from build123d import *

# Parameters (mm, degrees)
F0_R          = 7
F1_DEPTH      = 45
F4_DEPTH      = 10.5
F4_DEPTH_BACK = 13.5


with BuildPart() as f1:
    # F0 (on Front) → F1 (new body)
    with BuildSketch(Plane.XZ):
        with BuildLine():
            Line((-33.5, 28.5), (-40.5, 21.5))
            Line((-40.5, 21.5), (-40.5, -6.2290436868))
            Line((-40.5, -6.2290436868), (-32.4062898078, -13.2290436868))
            Line((-32.4062898078, -13.2290436868), (-4.3396635525, -13.2290436868))
            ThreePointArc((-4.3396635525, -13.2290436868), (-1.1020136669, -14.4188437946), (0.5947737455, -17.4219943993))
            ThreePointArc((0.5947737455, -17.4219943993), (2.6248372639, -24.3164832501), (6.2880673968, -30.5))
            Line((6.2880673968, -30.5), (14.5, -30.5))
            Line((14.5, -30.5), (43.5, 4.5))
            Line((43.5, 4.5), (43.5, 23.5))
            Line((43.5, 23.5), (35.5, 28.5))
            Line((35.5, 28.5), (6.5, 28.5))
            ThreePointArc((6.5, 28.5), (-0.361821699, 25.4052447636), (-7.8869164215, 25.2180111709))
            Line((-7.8869164215, 25.2180111709), (-26.5, 28.5))
            Line((-26.5, 28.5), (-33.5, 28.5))
        make_face()
        with Locations((-26.5, 0.7709563132)):
            Circle(F0_R, mode=Mode.SUBTRACT)
    extrude(amount=F1_DEPTH)

    # F3 (on offset) → F4 (cut, two sides)
    with BuildSketch(Plane.XZ.offset(22.5)) as f4_sk:
        with BuildLine():
            Line((35.5, 28.5), (11.6408265143, 28.5))
            ThreePointArc((11.6408265143, 28.5), (17.6190851715, 7.4683040803), (33.5571428571, -7.5))
            Line((33.5571428571, -7.5), (43.5, 4.5))
            Line((43.5, 4.5), (43.5, 23.5))
            Line((43.5, 23.5), (35.5, 28.5))
        make_face()
    extrude(amount=-F4_DEPTH, mode=Mode.SUBTRACT)
    extrude(f4_sk.sketch, amount=F4_DEPTH_BACK, mode=Mode.SUBTRACT)


solid = f1.part
The model under review builds one solid part; all positions refer to its coordinate system, in mm. A direction names the side the tool comes from. Coordinates: 2 decimals unless noted, no trailing zeros. Loops run counter-clockwise (first coordinate to the right, second up) from the corner with the lowest first, then second, coordinate; pieces in that order, holes last.
(1) Consider section C-C, the plane z = 16. Give the boundary of the cut face in (x, y), plus the area to 3 significant figures.
Determined:
outline: (-40.5, -45) - (43.5, -45) - (43.5, -36) - (13.69, -36) - (13.69, -12) - (43.5, -12) - (43.5, 0) - (-40.5, 0) - close
area: 3,060 mm2
(2) Wall thickness on L1, parallel to Z at x = -27, y = -2.5; L2, parallel to Y at x = 17.5, z = 9.5; L3, parallel to Z at x = -4, y = -7: over which ranges is each line inside the solid? List them lowest first.
Determined:
L1: z = -13.23 to -6.21, 7.75 to 28.5
L2: y = -45 to -36, -12 to 0
L3: z = -13.24 to 24.94
(3) Consider section A-A, the plane y = -4.5. Give the boundary of the cut face in (x, z).
Determined:
outline: (-40.5, -6.23) - (-32.41, -13.23) - (-4.34, -13.23) arc R5 cw to (0.59, -17.42) arc R29 ccw to (6.29, -30.5) - (14.5, -30.5) - (43.5, 4.5) - (43.5, 23.5) - (35.5, 28.5) - (6.5, 28.5) arc R19 cw to (-7.89, 25.22) - (-26.5, 28.5) - (-33.5, 28.5) - (-40.5, 21.5) - close; hole circle Ø14 at (-26.5, 0.77)
(4) Consider section D-D, the plane x = 26. Give the boundary of the cut face in (y, z).
Determined:
outline: (-45, -16.62) - (0, -16.62) - (0, 28.5) - (-12, 28.5) - (-12, -2.38) - (-36, -2.38) - (-36, 28.5) - (-45, 28.5) - close
(5) Insertion check: P1, Ø12, axis at y = -24.5, z = -24, coming from the -X side; P2, Ø10, axis at x = 35, y = -40, coming from the -Z side; P3, Ø10, axis at x = -24, y = -32.5, coming from the -Z side. Each pin has a flat end and moves straight along its axis. Give the tip position at first contact, or say it passes through.
Determined:
P1: stops at x = 0.7
P2: stops at z = -11.79
P3: stops at z = -13.23
(6) Draft analysis for pull direction X (two halves, no side actions). For faces 1 (the cylindrical face through (-1.14, -22.185, -14.387)), 2 (the cylindrical face through (-0.26, -22.18, 25.43)), 3 (the flat face through (43.5, -6, 14)), 4 (the flat face through (-30, -22, 28.5)), state which applies: +X half, -X half, draft (parallel to the pull), parting line (faces both ways), or undercut.
Determined:
face 1: -X half
face 2: undercut
face 3: +X half
face 4: draft
(7) Tool access review of faces 5 (the flat face through (39.556, -5.916, 25.965)), 6 (the flat face through (27, -36, 15)), 7 (the flat face through (-17.063, -22.185, 26.836)), 8 (the flat face through (-19, -22, -13.229)): name each direction out of +Z, -Z, +X, -X, +Y, -Y from which nothing blocks a thin tool from reaching the whole face with its end or side.
Determined:
face 5: +Z, +X, +Y, -Y
face 6: +Z, +X
face 7: +Z, +Y, -Y
face 8: -Z, -X, +Y, -Y
(8) Consider section B-B, the plane x = -20.5. Give the boundary of the cut face in (y, z), plus the area to 3 significant figures.
Determined:
outline: (-45, -13.23) - (0, -13.23) - (0, -2.83) - (-45, -2.83) - close; (-45, 4.38) - (0, 4.38) - (0, 27.44) - (-45, 27.44) - close
area: 1,510 mm2
